Part print with two shaded views. Sizes in mm from the minimum x, y, z corner. Round coordinates to 2 decimals unless told otherwise and drop trailing zeros. Order: outer loops, then holes, each group sorted by start corner. A loop starts at its lowest first (then second) coordinate and runs counter-clockwise, first axis right, second up. Notation, with made-up numbers: (-36, 30) - (4, 30) arc R22 cw to (4, 46) - close; hole circle Ø1 at (2, 22.5). An arc over 180 degrees is marked (long way). Write item = value, one per line.
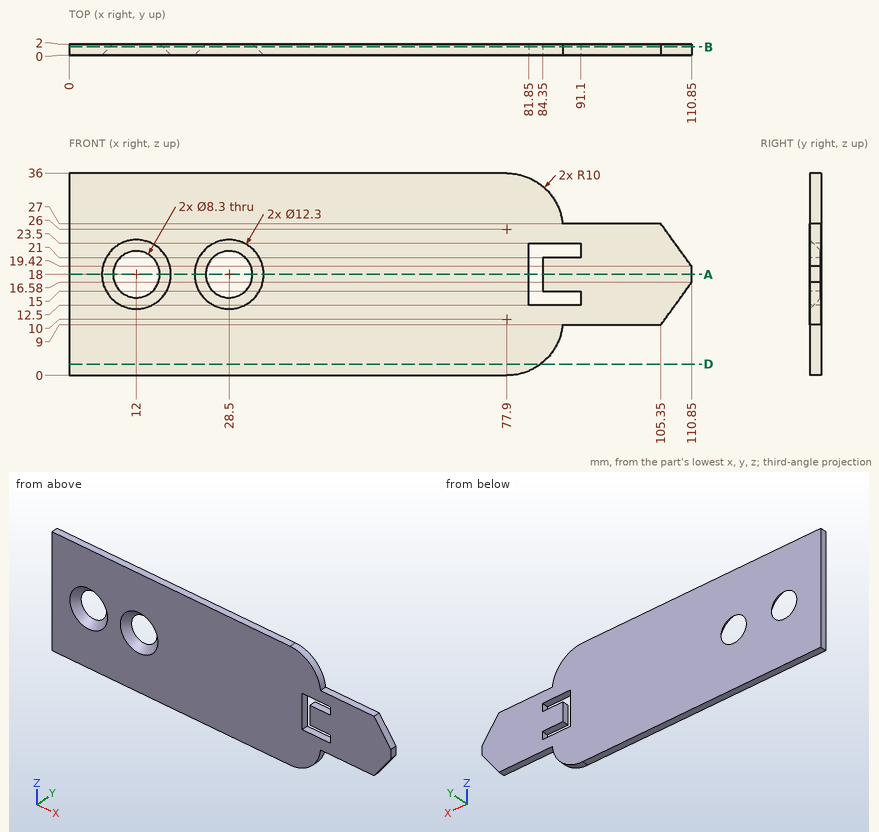
1) Cut at D-D (z = 2). Write the cut outline in (x, y), and give its area (3 significant figures).
Conclusion:
outline = (0, 0) - (83.9, 0) - (83.9, 2) - (0, 2) - close
area = 168 mm^2
2) Cut at A-A (z = 18). Give the number of separate pieces and of enclosed holes in the cut face, and give its area (4 significant figures).
Conclusion:
separate_pieces = 4
enclosed_holes = 0
area = 175.5 mm^2
3) Flat gauge pins, fed straight in: pin 1 Ø0.6 at (x, y) = (88.5, 1.5) entering from -Z; pin 2 Ø0.6 at (x, y) = (100, 1.5) entering from +Z. Where does each tip first touch, or does it go through?
Conclusion:
pin_1 = 9
pin_2 = 27
4) Cut at B-B (y = 1.5). Write the cut outline in (x, z).
Conclusion:
outline = (0, 0) - (77.9, 0) arc R10 ccw to (87.85, 9) - (105.35, 9) - (110.85, 16.58) - (110.85, 19.42) - (105.35, 27) - (87.85, 27) arc R10 ccw to (77.9, 36) - (0, 36) - close; hole circle Ø9.3 at (12, 18); hole circle Ø9.3 at (28.5, 18); hole (81.85, 12.5) - (91.1, 12.5) - (91.1, 15) - (84.35, 15) - (84.35, 21) - (91.1, 21) - (91.1, 23.5) - (81.85, 23.5) - close
5) Wall check: line 1 along X through (y, z) = (1.3, 20); line 2 along X through (y, z) = (1.6, 15.5); line 3 along Z through (x, y) = (84, 0.25). Give the ranges that are in metal, low to high.
Conclusion:
line_1 = 0 to 7.58, 16.42 to 24.08, 32.92 to 81.85, 84.35 to 110.43
line_2 = 0 to 8.2, 15.8 to 24.7, 32.3 to 81.85, 84.35 to 110.07
line_3 = 2.08 to 12.5, 23.5 to 33.92
